Design review of the part built by this model. Coordinates are the model's own, in mm. Give positions to 0.01 mm unless a question says otherwise; leave off trailing zeros. Write each loop counter-clockwise with the first axis right and the second up, starting at its lowest first coordinate (ties: lowest second). Pieces come first, ordered by that corner, then holes.
```python
from build123d import *

# Parameters (mm, degrees)
SKETCH1_R           = 330
SKETCH1_R_2         = 291
BOSS_EXTRUDE1_DEPTH = 5
SKETCH2_R           = 1.75
CUT_EXTRUDE1_DEPTH  = 6
CIRPATTERN1_COUNT   = 10


with BuildPart() as part:
    # Sketch1 → Boss-Extrude1 (new body)
    with BuildSketch(Plane(origin=(0, 0, 0), x_dir=(1, 0, 0), z_dir=(0, 1, 0))):
        Circle(SKETCH1_R)
        Circle(SKETCH1_R_2, mode=Mode.SUBTRACT)
    extrude(amount=-BOSS_EXTRUDE1_DEPTH)

    # Sketch2 → Cut-Extrude1 (cut, through all)
    with BuildSketch(Plane(origin=(0, 0, 0), x_dir=(1, 0, 0), z_dir=(0, 1, 0))):
        with Locations((5.238528177, -324.957778523)):
            Circle(SKETCH2_R)
        with Locations((94.250183284, -290.07223747)):
            Circle(SKETCH2_R)
        with Locations((175.273957266, -249.607772124)):
            Circle(SKETCH2_R)
    cut_extrude1 = extrude(amount=-CUT_EXTRUDE1_DEPTH, mode=Mode.SUBTRACT)

    # CirPattern1: Cut-Extrude1 ×10 about axis
    cirpattern1_axis = Axis((0, 0, 0), (0, 1, 0))
    for i in range(1, CIRPATTERN1_COUNT):
        add(cut_extrude1.rotate(cirpattern1_axis, i * 360 / CIRPATTERN1_COUNT), mode=Mode.SUBTRACT)


solid = part.part
```
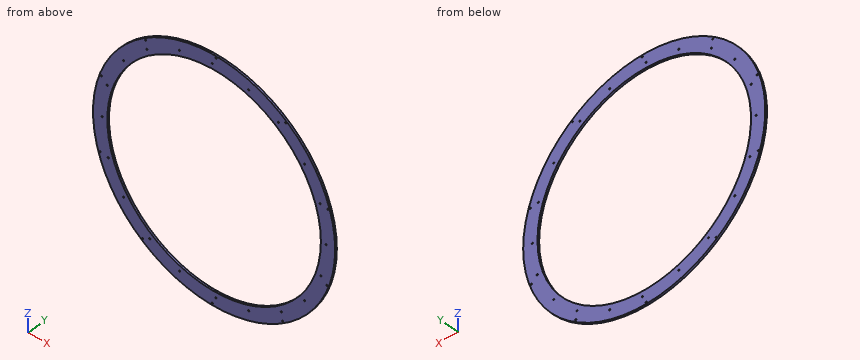
(1) Consider section C-C, the plane y = -3.9. Give the number of separate pieces and of enclosed holes in the cut face, then the cut area to 3 significant figures.
Resolved:
separate pieces: 1
enclosed holes: 31
area: 75,800 mm2
(2) Clearance check with flat-ended pins moving along their axes: P1, Ø1.5, axis at y = -2, z = -147, coming from the +X side; P2, Ø1, axis at x = -54.5, y = -3, coming from the -Z side. State where each tip first meets the part, or that it passes through.
Resolved:
P1: stops at x = 295.82
P2: stops at z = -325.55
(3) To check wall thickness, follow L1, parallel to Z at x = 1, y = -1.6; L2, parallel to X at y = -3.45, z = -243; L3, parallel to X at y = -2.7, z = 99.5. State the ranges of each line that lie inside material, in increasing order.
Resolved:
L1: z = -330 to -291, 291 to 330
L2: x = -223.27 to -160.1, 160.1 to 181.69, 184.77 to 223.27
L3: x = -314.64 to -273.46, 273.46 to 286.87, 290.16 to 314.64
(4) Consider section A-A, the plane z = 222. Give the boundary of the cut face in (x, y), then the cut area to 3 significant figures.
Resolved:
outline: (-244.16, -5) - (-188.14, -5) - (-188.14, 0) - (-244.16, 0) - close; (188.14, -5) - (244.16, -5) - (244.16, 0) - (188.14, 0) - close
area: 560 mm2
(5) Consider section B-B, the plane x = -73.5. Give the boundary of the cut face in (y, z).
Resolved:
outline: (-5, -321.71) - (0, -321.71) - (0, -281.56) - (-5, -281.56) - close; (-5, 281.56) - (0, 281.56) - (0, 321.71) - (-5, 321.71) - close
